Verification items for the finished model (mm, model axes). A direction names the side the tool comes from. Coordinates: 2 decimals unless noted, no trailing zeros. Write each loop counter-clockwise with the first axis right and the second up, starting at its lowest first coordinate (ties: lowest second). Pieces come first, ordered by that corner, then holes. Notation, with made-up numbers: M 10.5,77.5 L 28.5,77.5 A27 ccw 28.5,95.5 Z; hole C -30,48 d3. An arc over 180 degrees is marked long. Answer in a Markdown table with one row per item.
from build123d import *

# Parameters (mm, degrees)
F1_DEPTH = 25.4
F2_DEPTH = 127
F3_R     = 37.94188
F4_DEPTH = 50.8
F5_DEPTH = 127
F6_R     = 37.91738
F7_DEPTH = 50.8


with BuildPart() as f1:
    # F0 (on Front) → F1 (new body)
    with BuildSketch(Plane.XZ):
        Polygon((-24.067785, 0.039836), (-5.804424, 31.460671), (-23.883986, 62.987623), (-60.226907, 63.093739), (-78.490267, 31.672904), (-60.410706, 0.145952), align=None)
    extrude(amount=F1_DEPTH)

    # F1_face (on face) → F2 (join)
    with BuildSketch(Plane(origin=(-42.147346, 0, 31.566788), x_dir=(1, 0, 0), z_dir=(0, 1, 0))):
        Polygon((36.342922, 0.106116), (18.079561, 31.526951), (-18.26336, 31.420835), (-36.342922, -0.106116), (-18.079561, -31.526951), (18.26336, -31.420835), align=None)
        Polygon((18.079561, 31.526951), (36.342922, 0.106116), (18.26336, -31.420835), (-18.079561, -31.526951), (-36.342922, -0.106116), (-18.26336, 31.420835), align=None)
    extrude(amount=F2_DEPTH)

    # F3 (on Front) → F4 (join)
    with BuildSketch(Plane.XZ):
        with Locations((-43.137185, 32.617502)):
            Circle(F3_R)
    extrude(amount=F4_DEPTH)

    # F2_face (on face) → F5 (join)
    with BuildSketch(Plane(origin=(-42.147346, 127, 31.566788), x_dir=(1, 0, 0), z_dir=(0, 1, 0))):
        Polygon((18.26336, -31.420835), (36.342922, 0.106116), (18.079561, 31.526951), (-18.26336, 31.420835), (-36.342922, -0.106116), (-18.079561, -31.526951), align=None)
    extrude(amount=F5_DEPTH)

    # F6 (on Front) → F7 (join)
    with BuildSketch(Plane.XZ):
        with Locations((-43.654717, 32.360213)):
            Circle(F6_R)
    extrude(amount=F7_DEPTH)


solid = f1.part
1) Sectioned sample at C-C (z = 59). Record the cut outline in (x, y).
Response values:
| item | result |
|---|---|
| outline | M -70.64,-50.8 L -15.87,-50.8 L -15.87,0 L -21.6,0 L -21.6,254 L -62.61,254 L -62.61,0 L -70.64,0 Z |
2) Sectioned sample at A-A (y = 56.5). Record the cut outline in (x, z), then the cut area to 3 significant figures.
Response values:
| item | result |
|---|---|
| outline | M -78.49,31.67 L -60.41,0.15 L -24.07,0.04 L -5.8,31.46 L -23.88,62.99 L -60.23,63.09 Z |
| area | 3,430 mm² |
3) Thickness scan on L1, parallel to Z at x = -27, y = 175.5; L2, parallel to Z at x = -57.5, y = 65; L3, parallel to Y at x = -76, z = 24.5. Record the ranges inside material, lowest first. Write a range as [from, to].
Response values:
| item | result |
|---|---|
| L1 | z = [0.05, 63] |
| L2 | z = [0.14, 63.09] |
| L3 | y = [-50.8, 0] |
4) Sectioned sample at B-B (x = -17). Record the cut outline in (y, z), then the cut area to 3 significant figures.
Response values:
| item | result |
|---|---|
| outline | M -50.8,5.11 L 0,5.11 L 0,12.2 L 254,12.2 L 254,50.98 L 0,50.98 L 0,60.12 L -50.8,60.12 Z |
| area | 12,600 mm² |
5) Release check for a two-part mould opening along X. For faces 1 (the face through (-8.788, -25.044, 48.733)), 2 (the face through (-44, -50.8, 33)), 3 (the face through (-14.81, 125.22, 15.97)) record: +X half, -X half, draft (parallel to the pull), parting line (faces both ways), or undercut.
Response values:
| item | result |
|---|---|
| face 1 | parting line |
| face 2 | draft |
| face 3 | +X half |
6) Tool access check on faces 4 (the face through (-69.324, 125.222, 15.689)), 5 (the face through (-72, 0, 44)), 6 (the face through (-69.49, 125.22, 47.16)). Record the directions out of +Z, -Z, +X, -X, +Y, -Y that give a thin tool (end or side, any length) a straight path to the whole face; none if there is none.
Response values:
| item | result |
|---|---|
| face 4 | -Z, -X, +Y |
| face 5 | +Y |
| face 6 | +Z, -X, +Y |
7) Depth check by flat-ended pin: pin 1 (6 mm diameter, centred on x = -25, y = 173.5, fed in from -Z); pin 2 (5 mm diameter, centred on y = 191.5, z = 38, fed in from +X); pin 3 (4 mm diameter, centred on y = 136, z = 47.5, fed in from +X). Enter the tip coordinate at first touch or a pass-through.
Response values:
| item | result |
|---|---|
| pin 1 | stops at z = 0.04 |
| pin 2 | stops at x = -8.12 |
| pin 3 | stops at x = -13.86 |
